Could you check a few things on this drawing? It's one solid part, dimensions in mm from its lowest x, y, z. Give positions to 0.01 mm unless a question says otherwise; leave off trailing zeros. Order: outer loops, then holes, each group sorted by start corner. A loop starts at its lowest first (then second) coordinate and runs counter-clockwise, first axis right, second up. Notation, with made-up numbers: (30, 23.5) - (53, 23.5) arc R9 cw to (53, 37.5) - close; hole circle Ø11 at (27, -35.75). An arc over 180 degrees is marked (long way). Return JSON: item names as keys, results as strings.
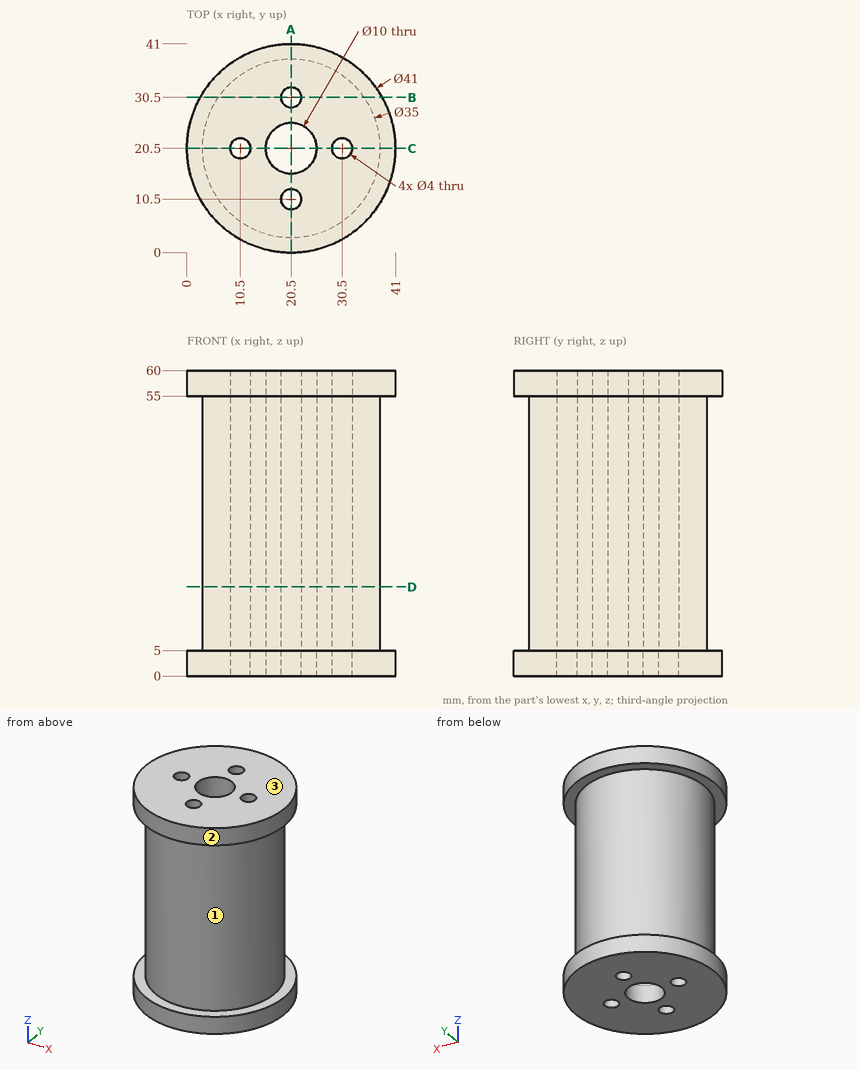
1. Suppose I cut it at A-A (x = 20.5). List the corners of the cut face in (y, z) for me, plus the area to 3 significant figures.
Checks:
{"outline": "(0, 0) - (8.5, 0) - (8.5, 60) - (0, 60) - (0, 55) - (3, 55) - (3, 5) - (0, 5) - close; (12.5, 0) - (15.5, 0) - (15.5, 60) - (12.5, 60) - close; (25.5, 0) - (28.5, 0) - (28.5, 60) - (25.5, 60) - close; (32.5, 0) - (41, 0) - (41, 5) - (38, 5) - (38, 55) - (41, 55) - (41, 60) - (32.5, 60) - close", "area": "1,080 mm^2"}
2. Suppose I cut it at B-B (y = 30.5). List the corners of the cut face in (x, z) for me.
Checks:
{"outline": "(2.6, 0) - (18.5, 0) - (18.5, 60) - (2.6, 60) - (2.6, 55) - (6.14, 55) - (6.14, 5) - (2.6, 5) - close; (22.5, 0) - (38.4, 0) - (38.4, 5) - (34.86, 5) - (34.86, 55) - (38.4, 55) - (38.4, 60) - (22.5, 60) - close"}
3. Thinking about a two-plate mould opening in Z: for the marked faces 1, 2 and 3, which applies, +Z half, -Z half, draft (parallel to the pull), parting line (faces both ways), or undercut?
Checks:
{"face 1": "undercut", "face 2": "draft", "face 3": "+Z half"}
4. For pin 1 Ø5 at (y, z) = (6.5, 11) entering from +X; pin 2 Ø3 at (x, z) = (8, 19) entering from +Y; pin 3 Ø2 at (y, z) = (32.5, 48.5) entering from -X, each with a flat end and sliding along its axis, tell me the tip position at first contact or that it passes through.
Checks:
{"pin 1": "x = 33.69", "pin 2": "y = 34.11", "pin 3": "x = 6.89"}
5. If I drill on L1, parallel to Y at x = 20.5, z = 35.5; L2, parallel to Z at x = 5.5, y = 32.5; L3, parallel to Y at x = 20.5, z = 3.9, over which ranges is the centre line in solid material (lowest first)? Write a range as [from, to].
Checks:
{"L1": "[3, 8.5], [12.5, 15.5], [25.5, 28.5], [32.5, 38]", "L2": "[0, 5], [55, 60]", "L3": "[0, 8.5], [12.5, 15.5], [25.5, 28.5], [32.5, 41]"}
6. Suppose I cut it at D-D (z = 17.5). List the corners of the cut face in (x, y) for me.
Checks:
{"outline": "circle Ø35 at (20.5, 20.5); hole circle Ø4 at (10.5, 20.5); hole circle Ø10 at (20.5, 20.5); hole circle Ø4 at (20.5, 10.5); hole circle Ø4 at (20.5, 30.5); hole circle Ø4 at (30.5, 20.5)"}
